The listing builds one solid part. Answer for the finished solid, in the listing's coordinates (mm). A direction names the side the tool comes from. Give positions to 0.01 mm unless a question says otherwise; leave off trailing zeros. Loops run counter-clockwise (first coordinate to the right, second up) from the corner with the lowest first, then second, coordinate; pieces in that order, holes last. Notation, with made-up numbers: M 29,-14.75 L 75,-14.75 A19 cw 75,10.25 Z; hole C 8,-3 d10. An arc over 180 degrees is marked long. Return JSON: item names as keys, results as strings.
from build123d import *

# Parameters (mm, degrees)
SKETCH_R     = 1.8
PAD_DEPTH    = 10
SKETCH001_R  = 1.8
POCKET_DEPTH = 133.001


with BuildPart() as part:
    # Sketch → Pad (new body)
    with BuildSketch(Plane.XY):
        with BuildLine():
            ThreePointArc((-60.5, 20.182105), (-59.5, 11.7), (-58.5, 20.182105))
            Line((-58.5, 26), (-58.5, 20.182105))
            Line((-58.5, 26), (-52.5, 26))
            Line((-52.5, 26), (-52.5, 6))
            Line((-52.5, 6), (52.5, 6))
            Line((52.5, 6), (52.5, 26))
            Line((52.5, 26), (58.484608, 26))
            Line((58.484608, 20.178394), (58.484608, 26))
            ThreePointArc((58.484608, 20.178394), (59.515826, 11.700029), (60.484608, 20.185755))
            Line((60.484608, 26), (60.484608, 20.185755))
            Line((60.484608, 26), (66.5, 26))
            Line((66.5, 26), (66.5, 0))
            Line((66.5, 0), (-66.5, 0))
            Line((-66.5, 0), (-66.5, 26))
            Line((-66.5, 26), (-60.5, 26))
            Line((-60.5, 20.182105), (-60.5, 26))
        make_face()
        with Locations((-59.5, 5)):
            Circle(SKETCH_R, mode=Mode.SUBTRACT)
        with Locations((59.5, 5)):
            Circle(SKETCH_R, mode=Mode.SUBTRACT)
    extrude(amount=PAD_DEPTH)

    # Sketch001 → Pocket (cut, through all)
    with BuildSketch(Plane(origin=(-66.5, 0, 0), x_dir=(0, -1, 0), z_dir=(-1, 0, 0))):
        with Locations((-22.5, 5)):
            Circle(SKETCH001_R)
    extrude(amount=-POCKET_DEPTH, mode=Mode.SUBTRACT)


solid = part.part
(1) Determine the mould class of faces 1 (the flat face through (58.485, 24.3, 3.8)), 2 (the cylindrical face through (-55.542, 20.837, 4.311)), 3 (the flat face through (66.5, 13, 5)) for opening direction X: released by +X, released by -X, zero draft, split by the parting line, or undercut.
Values follow:
{"face 1": "undercut", "face 2": "zero draft", "face 3": "released by +X"}
(2) Straight lines are drawn through the part: line 1 along Z through (x, y) = (-54.8, 22.5); line 2 along X through (y, z) = (11.25, 3); line 3 along Y through (x, z) = (59.5, 6). For each, find the intervals that lie inside material, in ascending order.
Values follow:
{"line 1": "0 to 3.2, 6.8 to 10", "line 2": "-66.5 to -52.5, 52.5 to 66.5", "line 3": "0 to 3.2, 6.8 to 11.7"}
(3) A tool of negligible diameter and unlimited length cuts with its end or side. For faces 4 (the flat face through (55, 26, 5)), 5 (the flat face through (-58.5, 24.4, 3.8)), from which of +Z, -Z, +X, -X, +Y, -Y can it reach the whole face along a straight path? Write none if from no direction.
Values follow:
{"face 4": "+Z, -Z, +X, -X, +Y", "face 5": "+Z, -Z, +Y"}
(4) The part is cut by section B-B (y = 16). Determine the outline of the cut face in (x, z).
Values follow:
{"outline": "M -66.5,0 L -63.8,0 L -63.8,10 L -66.5,10 Z; M -55.2,0 L -52.5,0 L -52.5,10 L -55.2,10 Z; M 52.5,0 L 55.2,0 L 55.2,10 L 52.5,10 Z; M 63.8,0 L 66.5,0 L 66.5,10 L 63.8,10 Z"}
(5) The part is cut by section A-A (z = 5). Give the number of separate pieces and of enclosed holes in the cut face, and give its area (3 significant figures).
Values follow:
{"separate pieces": "5", "enclosed holes": "2", "area": "1,110 mm²"}
(6) Given pin 1 (1.5 mm diameter, centred on x = -7.5, z = 8.5, fed in from +Y); pin 2 (7 mm diameter, centred on x = 59.5, y = 16, fed in from -Z), each flat-ended and moving along its own axis, determine where each tip first touches the part or whether it passes through.
Values follow:
{"pin 1": "y = 6", "pin 2": "through"}
(7) The part is cut by section D-D (x = 0.5). Determine the outline of the cut face in (y, z).
Values follow:
{"outline": "M 0,0 L 6,0 L 6,10 L 0,10 Z"}
